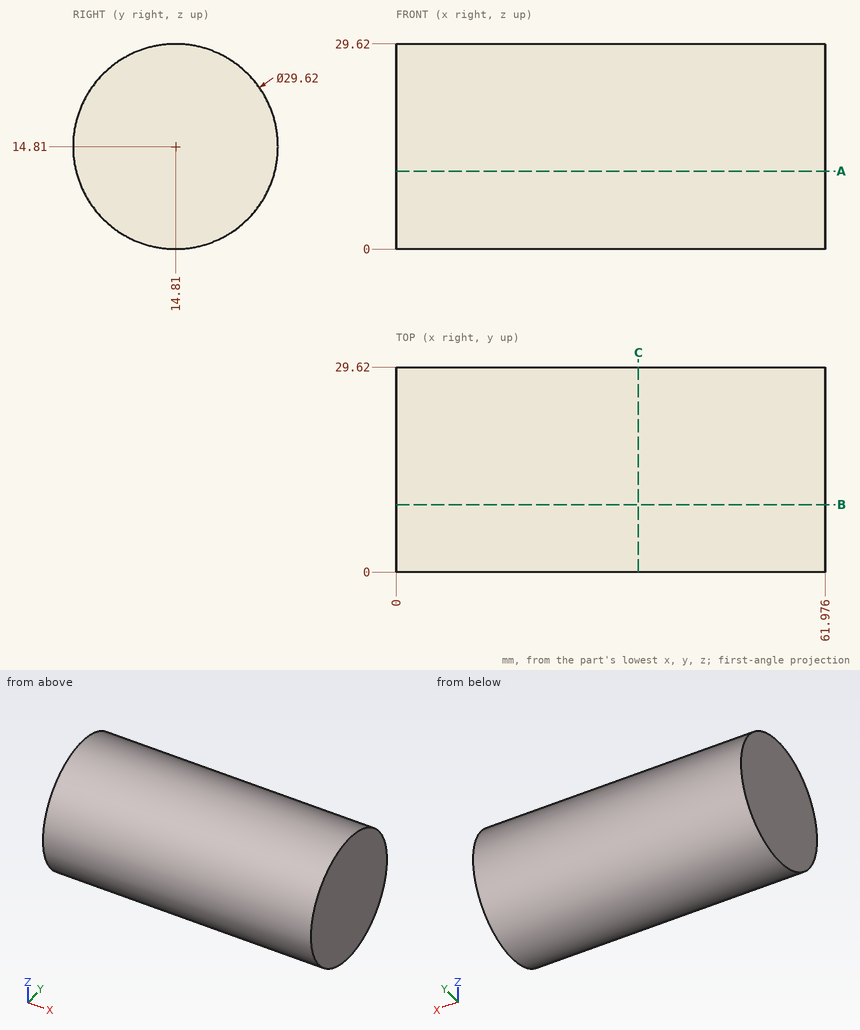
Study the drawing (mm; zero at the part's minimum x, y, z) and answer. Coordinates: 2 decimals unless noted, no trailing zeros. Write each loop counter-clockwise with the first axis right and the second up, starting at its lowest first coordinate (ties: lowest second). Pieces come first, ordered by that corner, then holes.
Q1. A cutting plane is placed at A-A, the plane z = 11.25. Give the vertices of the cut face in (x, y).
Q2. A cutting plane is placed at C-C, the plane x = 35. Give the vertices of the cut face in (y, z).
Q3. Find the intervals of material crossed by line 1 (Z direction, x = 56, y = 15); line 2 (Z direction, x = 46, y = 7.25) (1 decimal); line 3 (Y direction, x = 35, z = 12.5), in increasing order.
Q4. Each of these flat-tipped pins is pushed along its axis until it touches: pin 1 Ø8 at (x, z) = (34, 22.5) entering from -Y; pin 2 Ø3 at (x, y) = (17.5, 21) entering from +Z; pin 3 Ø1.5 at (x, y) = (34, 3.5) entering from -Z. Where does it stop, or does it pass through?
Q5. A cutting plane is placed at B-B, the plane y = 9.75. Give the vertices of the cut face in (x, z), then the cut area to 3 significant figures.
Findings below:
1. outline: (0, 0.43) - (61.98, 0.43) - (61.98, 29.19) - (0, 29.19) - close
2. outline: circle Ø29.62 at (14.81, 14.81)
3. line 1: z = 0 to 29.62
3. line 2: z = 2.1 to 27.5
3. line 3: y = 0.18 to 29.44
4. pin 1: stops at y = 0.47
4. pin 2: stops at z = 28.86
4. pin 3: stops at z = 4.43
5. outline: (0, 0.89) - (61.98, 0.89) - (61.98, 28.73) - (0, 28.73) - close
5. area: 1,730 mm2
